Check sheet for the drawn part. Datum: minimum x, y, z corner. Units: mm. A direction names the side the tool comes from. Round coordinates to 2 decimals unless told otherwise and drop trailing zeros. Write each loop counter-clockwise with the first axis right and the second up, starting at its lowest first coordinate (ties: lowest second). Pieces come first, ordered by that corner, then holes.
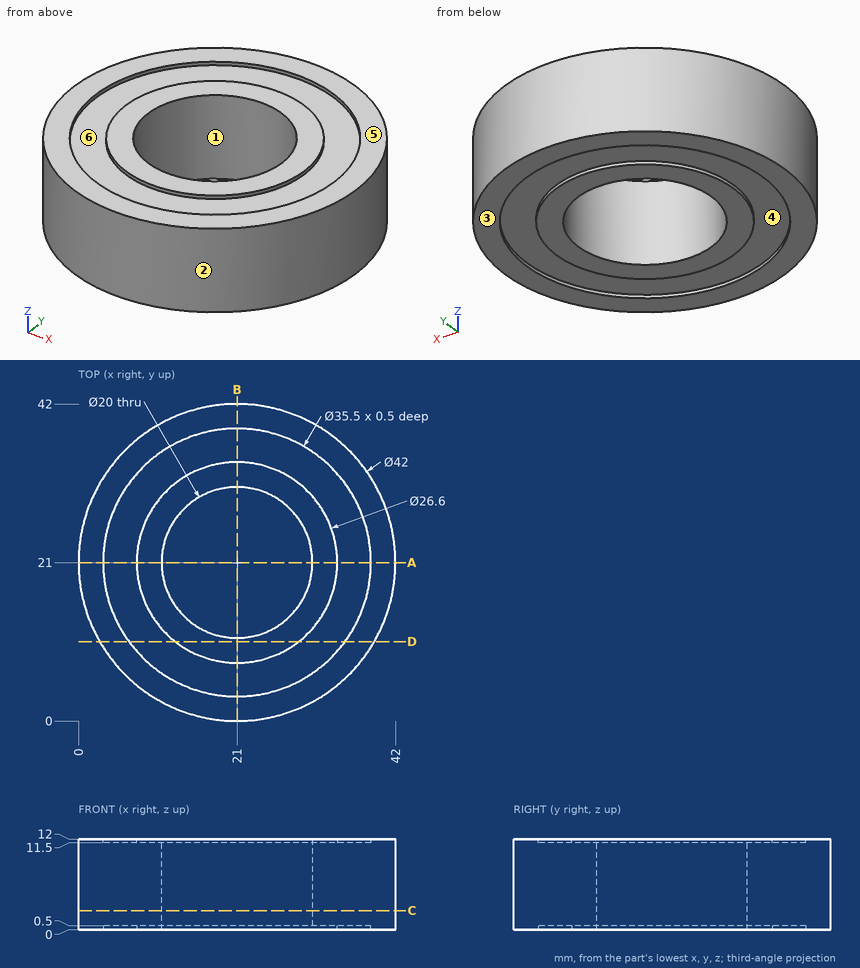
1. Set-up check for the marked faces 4, 5 and 6: record each of +Z, -Z, +X, -X, +Y, -Y from which the full face is reachable in a straight line by a thin tool's end or side.
2. Release check for a two-part mould opening along X. For the marked faces 1, 2 and 3 record: released by +X, released by -X, zero draft, split by the parting line, or undercut.
3. Sectioned sample at A-A, the plane y = 21. Enter the section's corners in (x, z).
4. Scan lines: line 1 along Y through (x, z) = (21, 11.7); line 2 along Z through (x, y) = (8, 17); line 3 along Y through (x, z) = (21, 6). Record each from-to range of solid material in increasing order.
5. Sectioned sample at C-C, the plane z = 2.5. Enter the section's corners in (x, y).
6. Go/stop test with flat-tipped pins: pin 1 (12 mm diameter, centred on x = 19.5, y = 24.5, fed in from -Z); pin 2 (1 mm diameter, centred on x = 17, z = 7, fed in from +Y); pin 3 (3 mm diameter, centred on x = 8, z = 8, fed in from -Y); pin 4 (2 mm diameter, centred on x = 6.5, y = 27, fed in from -Z). Record where each tip stops, or that it passes through.
7. Sectioned sample at D-D, the plane y = 10.5. Enter the section's corners in (x, z).
Computed values:
1. face 4: -Z
1. face 5: +Z, +X, -X, +Y, -Y
1. face 6: +Z
2. face 1: undercut
2. face 2: split by the parting line
2. face 3: zero draft
3. outline: (0, 0) - (3.25, 0) - (3.25, 0.5) - (7.7, 0.5) - (7.7, 0) - (11, 0) - (11, 12) - (7.7, 12) - (7.7, 11.5) - (3.25, 11.5) - (3.25, 12) - (0, 12) - close; (31, 0) - (34.3, 0) - (34.3, 0.5) - (38.75, 0.5) - (38.75, 0) - (42, 0) - (42, 12) - (38.75, 12) - (38.75, 11.5) - (34.3, 11.5) - (34.3, 12) - (31, 12) - close
4. line 1: y = 0 to 3.25, 7.7 to 11, 31 to 34.3, 38.75 to 42
4. line 2: z = 0.5 to 11.5
4. line 3: y = 0 to 11, 31 to 42
5. outline: circle Ø42 at (21, 21); hole circle Ø20 at (21, 21)
6. pin 1: passes through
6. pin 2: stops at y = 41.71
6. pin 3: stops at y = 3.43
6. pin 4: stops at z = 0.5
7. outline: (2.81, 0) - (6.69, 0) - (6.69, 0.5) - (12.84, 0.5) - (12.84, 0) - (29.16, 0) - (29.16, 0.5) - (35.31, 0.5) - (35.31, 0) - (39.19, 0) - (39.19, 12) - (35.31, 12) - (35.31, 11.5) - (29.16, 11.5) - (29.16, 12) - (12.84, 12) - (12.84, 11.5) - (6.69, 11.5) - (6.69, 12) - (2.81, 12) - close
